```python
from build123d import *

# Parameters (mm, degrees)
SKETCH1_W           = 38.1
SKETCH1_H           = 76.2
BOSS_EXTRUDE1_DEPTH = 41.275
SKETCH2_W           = 38.1
SKETCH2_H           = 28.575
CUT_EXTRUDE1_DEPTH  = 69.85
SKETCH3_R           = 14.2875
CUT_EXTRUDE2_DEPTH  = 60.313894873
FILLET1_R           = 3.175


with BuildPart() as part:
    # Sketch1 → Boss-Extrude1 (new body)
    with BuildSketch(Plane(origin=(0, 0, 0), x_dir=(1, 0, 0), z_dir=(0, 1, 0))):
        Rectangle(SKETCH1_W, SKETCH1_H)
    extrude(amount=BOSS_EXTRUDE1_DEPTH)

    # Sketch2 → Cut-Extrude1 (cut)
    with BuildSketch(Plane.XY.offset(38.1)):
        with Locations((0, 20.6375)):
            Rectangle(SKETCH2_W, SKETCH2_H)
    extrude(amount=-CUT_EXTRUDE1_DEPTH, mode=Mode.SUBTRACT)

    # Sketch3 → Cut-Extrude2 (cut, through all)
    # profile 1 of 2: a face of its own
    with BuildSketch(Plane(origin=(0, 41.275, 0), x_dir=(1, 0, 0), z_dir=(0, 1, 0))):
        with Locations(Location((0, -19.05, 0), (0, 0, 270))):
            Circle(SKETCH3_R)
        Polygon((7.332348419, -19.05), (3.666174209, -12.7), (-3.666174209, -12.7), (-7.332348419, -19.05), (-3.666174209, -25.4), (3.666174209, -25.4), align=None, mode=Mode.SUBTRACT)
    # profile 2 of 2: a face of its own
    with BuildSketch(Plane(origin=(0, 41.275, 0), x_dir=(1, 0, 0), z_dir=(0, 1, 0))):
        Polygon((3.666174209, -25.4), (7.332348419, -19.05), (3.666174209, -12.7), (-3.666174209, -12.7), (-7.332348419, -19.05), (-3.666174209, -25.4), align=None)
    extrude(amount=-CUT_EXTRUDE2_DEPTH, mode=Mode.SUBTRACT)

    # Fillet1
    fillet1_edges = [part.edges().sort_by_distance(p)[0] for p in [
        (0, 41.275, 38.1),
        (0, 0, -38.1),
        (0, 0, 38.1),
        (0, 6.35, 38.1),
        (0, 6.35, -31.75),
        (0, 34.925, -31.75),
        (0, 34.925, 38.1),
        (0, 41.275, -38.1),
        (-19.05, 0, 0),
    ]]
    fillet(fillet1_edges, radius=FILLET1_R - 0.0001)  # a hair under: the kernel refuses the full size


solid = part.part
```
Build history of the part. All positions in model axes, mm. A direction names the side the tool comes from. Round coordinates to 2 decimals unless told otherwise and drop trailing zeros. Loops run counter-clockwise (first coordinate to the right, second up) from the corner with the lowest first, then second, coordinate; pieces in that order, holes last. Notation, with made-up numbers: M 73.25,86.25 L 127.25,86.25 A26 ccw 127.25,122.25 Z; hole C -34,0 d7. An arc over 180 degrees is marked long. Answer as CSV lines item,"result".
1. Cut at D-D on z = -19.5. Write the cut outline in (x, y) (3 decimals).
Resolved:
outline,"M -19.05,3.175 A3.175 ccw -15.875,0 L 19.05,0 L 19.05,6.35 L -19.05,6.35 Z; M -19.05,34.925 L 19.05,34.925 L 19.05,41.275 L -19.05,41.275 Z"
2. 3-axis set-ups, long thin cutter, end or side, ignore diameter. For faces 4 (the cylindrical face through (0.267, 40.32, -37.195)), 5 (the cylindrical face through (0.27, 5.44, 37.15)): which of +Z, -Z, +X, -X, +Y, -Y reach the whole face in a straight line?
Resolved:
face 4,"-Z, +X, -X, +Y"
face 5,"+Z, +X, -X"
3. Cut at A-A on x = 0. Count the separate pieces of the cut face and the enclosed holes in it, then the cut area to 3 significant figures.
Resolved:
separate pieces,"3"
enclosed holes,"0"
area,"778 mm²"
4. Two-plate mould, pull along Z, no slides. Class faces 1 (the flat face through (0, 21, -31.75)), 2 (the flat face through (0, 6.35, -3)), 3 (the cylindrical face through (-5.47, 38.14, 32.25)): released by +Z, released by -Z, zero draft, split by the parting line, or undercut.
Resolved:
face 1,"released by +Z"
face 2,"zero draft"
face 3,"undercut"
5. Flat gauge pins, fed straight in: P1, Ø11.5, axis at x = 2, z = 15.5, coming from the +Y side; P2, Ø11, axis at x = -9, y = 25.5, coming from the +Z side. Where does each tip first touch, or does it go through?
Resolved:
P1,"passes through"
P2,"stops at z = -31.75"
6. Wall check: probe 1 along Y at (x, z) = (15, -1.5) (3 decimals); probe 2 along X at (y, z) = (37, 19); probe 3 along X at (y, z) = (2, 19). Give the ranges that are in metal, low to high. Write a range as [from, to].
Resolved:
probe 1,"y = [0, 6.35], [34.925, 41.275]"
probe 2,"x = [-19.05, -14.29], [14.29, 19.05]"
probe 3,"x = [-18.82, -14.29], [14.29, 19.05]"
